CAD build for the part. Positions are in the model's coordinates, mm. A direction names the side the tool comes from. Round coordinates to 2 decimals unless told otherwise and drop trailing zeros. Order: outer loops, then holes, each group sorted by start corner. A loop starts at its lowest first (then second) coordinate and runs counter-clockwise, first axis right, second up. Notation, with made-up numbers: (-30, 73.5) - (29, 73.5) arc R20 ccw to (29, 105.5) - close; hole circle Ø4 at (35.5, 84). An arc over 180 degrees is marked (long way). Use one line per item in the form item = value. Start each with the question number.
from build123d import *

# Parameters (mm, degrees)
BOSS_EXTRUDE1_DEPTH     = 35
SKETCH3_R               = 2.6
CUT_EXTRUDE1_DEPTH      = 58.716981903
FILLET1_DEPTH           = 35
SKETCH5_R               = 2.3
CUT_EXTRUDE3_DEPTH      = 10
SKETCH7_W               = 40
SKETCH7_H               = 1.4
SKETCH7_H_2             = 10
BOSS_EXTRUDE2_DEPTH     = 5
CUT_EXTRUDE2_DEPTH      = 70.641941558
CUT_EXTRUDE2_DEPTH_BACK = 12
SKETCH4_R               = 2.2
CUT_EXTRUDE4_DEPTH      = 60.843546189
FILLET2_R               = 0.75
BOSS_EXTRUDE3_DEPTH     = 40
FILLET3_R               = 0.75
FILLET4_R               = 0.25
FILLET5_R               = 5


with BuildPart() as part:
    # Sketch1 → Boss-Extrude1 (new body)
    with BuildSketch(Plane(origin=(0, 0, 0), x_dir=(1, 0, 0), z_dir=(0, 1, 0))):
        Polygon((0, 22.5), (0, -22.5), (30, -22.5), (30, 19.5), (40, 19.5), (40, 22.5), align=None)
    extrude(amount=BOSS_EXTRUDE1_DEPTH)

    # Sketch3 → Cut-Extrude1 (cut, through all)
    with BuildSketch(Plane.ZY):
        with Locations((3.62, 17.5)):
            Circle(SKETCH3_R)
    extrude(amount=-CUT_EXTRUDE1_DEPTH, mode=Mode.SUBTRACT)

    # Fillet1: read off the stored shape, not the designer's step
    # Fillet1 outline → Fillet1 (add)
    with BuildSketch(Plane(origin=(0, 0, 0), x_dir=(1, 0, 0), z_dir=(0, 1, 0))):
        with BuildLine():
            Line((30, 19.5), (30, 4.301315846))
            add(Edge.make_bspline(
                [(30, 4.301315846), (30, 16.210241525), (40, 19.5)],
                knots=[0, 0, 0, 1, 1, 1], degree=2, weights=[1, 0.810092587, 1]))
            Line((40, 19.5), (30, 19.5))
        make_face()
    extrude(amount=FILLET1_DEPTH)

    # Sketch5 → Cut-Extrude3 (cut)
    with BuildSketch(Plane.XY.offset(22.5)):
        with Locations((5, 30)):
            Circle(SKETCH5_R)
        with Locations((5, 5)):
            Circle(SKETCH5_R)
        with Locations((25, 5)):
            Circle(SKETCH5_R)
        with Locations((25, 30)):
            Circle(SKETCH5_R)
    extrude(amount=-CUT_EXTRUDE3_DEPTH, mode=Mode.SUBTRACT)

    # Sketch7 → Boss-Extrude2 (add)
    with BuildSketch(Plane(origin=(0, 0, -22.5), x_dir=(-1, 0, 0), z_dir=(0, 0, -1))):
        with Locations((-20, 34.3)):
            Rectangle(SKETCH7_W, SKETCH7_H)
        with Locations((-20, 15.30039382)):
            Rectangle(SKETCH7_W, SKETCH7_H_2)
    extrude(amount=BOSS_EXTRUDE2_DEPTH)

    # Sketch4 → Cut-Extrude2 (cut, two sides: drawn at the far end of the back side and taken through both)
    with BuildSketch(Plane(origin=(0, 0, -22.5), x_dir=(-1, 0, 0), z_dir=(0, 0, -1)).offset(-CUT_EXTRUDE2_DEPTH_BACK)):
        with Locations((-5.5, 17.5)):
            Circle(SKETCH4_R)
    extrude(amount=CUT_EXTRUDE2_DEPTH + CUT_EXTRUDE2_DEPTH_BACK, mode=Mode.SUBTRACT)

    # Sketch9 → Cut-Extrude4 (cut, through all)
    with BuildSketch(Plane(origin=(40, 0, 0), x_dir=(0, 0, -1), z_dir=(1, 0, 0))):
        with BuildLine():
            Line((27.5, 20.30039382), (24.3, 20.30039382))
            Line((24.3, 20.30039382), (24.3, 16.5))
            ThreePointArc((24.3, 16.5), (25.182933063, 13.75773816), (27.5, 12.04578851))
            Line((27.5, 12.04578851), (27.5, 20.30039382))
        make_face()
    extrude(amount=-CUT_EXTRUDE4_DEPTH, mode=Mode.SUBTRACT)

    # Fillet2
    # the kernel refuses this fillet: 0.75 mm, written as the material it takes off along each edge
    with BuildSketch(Plane(origin=(41.875, 20.30039382, -24.3), x_dir=(0, 0, 1), z_dir=(-1, 0, 0))) as fillet2_piece_1:
        with BuildLine():
            CenterArc((FILLET2_R, -FILLET2_R), FILLET2_R, 90, 90)
            Line((0, -FILLET2_R), (0, 0))
            Line((0, 0), (FILLET2_R, 0))
        make_face()
    extrude(amount=43.75, mode=Mode.SUBTRACT)

    # Sketch10 → Boss-Extrude3 (add, through all)
    with BuildSketch(Plane(origin=(40, 0, 0), x_dir=(0, 0, -1), z_dir=(1, 0, 0))):
        with BuildLine():
            Line((30.420638784, 11.76058351), (29.969418861, 11.76058351))
            add(Edge.make_bspline(
                [(27.5, 12.04578851), (28.285278796, 11.781338069), (29.10521732, 11.76058351), (29.969418861, 11.76058351)],
                knots=[0, 0, 0, 0, 1, 1, 1, 1], degree=3))
            Line((27.5, 12.04578851), (27.5, 10.30039382))
            Line((27.5, 10.30039382), (30.420638784, 10.30039382))
            ThreePointArc((30.420638784, 10.30039382), (32.925002128, 10.70728085), (35.171736316, 11.886084613))
            ThreePointArc((35.171736316, 11.886084613), (35.316984097, 12.908327269), (34.294741441, 13.05357505))
            ThreePointArc((34.294741441, 13.05357505), (32.462727085, 12.092364139), (30.420638784, 11.76058351))
        make_face()
    extrude(amount=-BOSS_EXTRUDE3_DEPTH)

    # Fillet3
    # the kernel refuses this fillet: 0.75 mm, written as the material it adds along each edge
    with BuildSketch(Plane(origin=(40, 20.30039382, -22.5), x_dir=(0, 1, 0), z_dir=(-1, 0, 0))) as fillet3_piece_1:
        with BuildLine():
            CenterArc((FILLET3_R, FILLET3_R), FILLET3_R, 180, 90)
            Line((0, FILLET3_R), (0, 0))
            Line((0, 0), (FILLET3_R, 0))
        make_face()
    extrude(amount=40)
    # the kernel refuses this fillet: 0.75 mm, written as the material it takes off along each edge
    with BuildSketch(Plane(origin=(41.875, 35, -27.5), x_dir=(0, -1, 0), z_dir=(-1, 0, 0))) as fillet3_2_piece_1:
        with BuildLine():
            CenterArc((FILLET3_R, FILLET3_R), FILLET3_R, 180, 90)
            Line((0, FILLET3_R), (0, 0))
            Line((0, 0), (FILLET3_R, 0))
        make_face()
    extrude(amount=43.75, mode=Mode.SUBTRACT)
    with BuildSketch(Plane(origin=(-1.875, 33.6, -27.5), x_dir=(0, 0, 1), z_dir=(1, 0, 0))) as fillet3_2_piece_2:
        with BuildLine():
            CenterArc((FILLET3_R, -FILLET3_R), FILLET3_R, 90, 90)
            Line((0, -FILLET3_R), (0, 0))
            Line((0, 0), (FILLET3_R, 0))
        make_face()
    extrude(amount=43.75, mode=Mode.SUBTRACT)

    # Fillet4
    fillet4_edges = [part.edges().sort_by_distance(p)[0] for p in [
        (20, 33.6, -22.5),
    ]]
    fillet(fillet4_edges, radius=FILLET4_R)

    # Fillet5
    fillet5_edges = [part.edges().sort_by_distance(p)[0] for p in [
        (20, 10.30039382, -22.5),
    ]]
    fillet(fillet5_edges, radius=FILLET5_R)


solid = part.part
(1) Which spindle directions (+Z, -Z, +X, -X, +Y, -Y) get a long thin tool onto all of the face, cutting with end or side? Do faces 4 (the flat face through (6, 18, -10.5)), 5 (the flat face through (25, 30, 12.5)), 6 (the cylindrical face through (20.28, 13.79, -25.16)), 7 (the cylindrical face through (20.3, 10.7, -32.9)), 8 (the flat face through (20, 27, -22.5)). Say none if no direction does.
(2) Slice it at A-A (z = 3.62). Give the cut face in (x, y).
(3) Wall check: line 1 (Y direction, x = 5, z = 18); line 2 (X direction, y = 17.5, z = -20.5); line 3 (Y direction, x = 19.5, z = 3.62). Give the ranges that are in metal, low to high. Write a range as [from, to].
(4) Slice it at B-B (z = 17.5). Give the cut face in (x, y), and give its area (3 significant figures).
(5) Mould opens along Y. For faces 1 (the flat face through (40, 18, -22)), 2 (the cylindrical face through (27.125, 4.119, 17.57)), 3 (the cylindrical face through (19.72, 8.8, -23.93)) say: pulls with the +Y half, pulls with the -Y half, needs draft (parallel to the pull), parting line crosses it, or undercut.
(6) Flat gauge pins, fed straight in: P1, Ø3.5, axis at x = 5, y = 30, coming from the +Z side; P2, Ø7.5, axis at x = 5, y = 5, coming from the -Z side; P3, Ø4, axis at x = 27, y = 25, coming from the -Z side. Where does each tip first touch, or does it go through?
Results list:
q1.face_4 = -Z
q1.face_5 = +Z
q1.face_6 = +X, -X
q1.face_7 = -Z, +X, -X, -Y
q1.face_8 = -Z, +X, -X
q2.outline = (0, 0) - (30, 0) - (30, 14.9) - (0, 14.9) - close; (0, 20.1) - (30, 20.1) - (30, 35) - (0, 35) - close
q3.line_1 = [0, 2.7], [7.3, 27.7], [32.3, 35]
q3.line_2 = [0, 3.3], [7.7, 40]
q3.line_3 = [0, 14.9], [20.1, 35]
q4.outline = (0, 0) - (30, 0) - (30, 35) - (0, 35) - close; hole circle Ø4.6 at (5, 5); hole circle Ø4.6 at (5, 30); hole circle Ø4.6 at (25, 5); hole circle Ø4.6 at (25, 30)
q4.area = 984 mm²
q5.face_1 = needs draft
q5.face_2 = undercut
q5.face_3 = pulls with the -Y half
q6.P1 = 12.5
q6.P2 = -23.88
q6.P3 = -22.5
